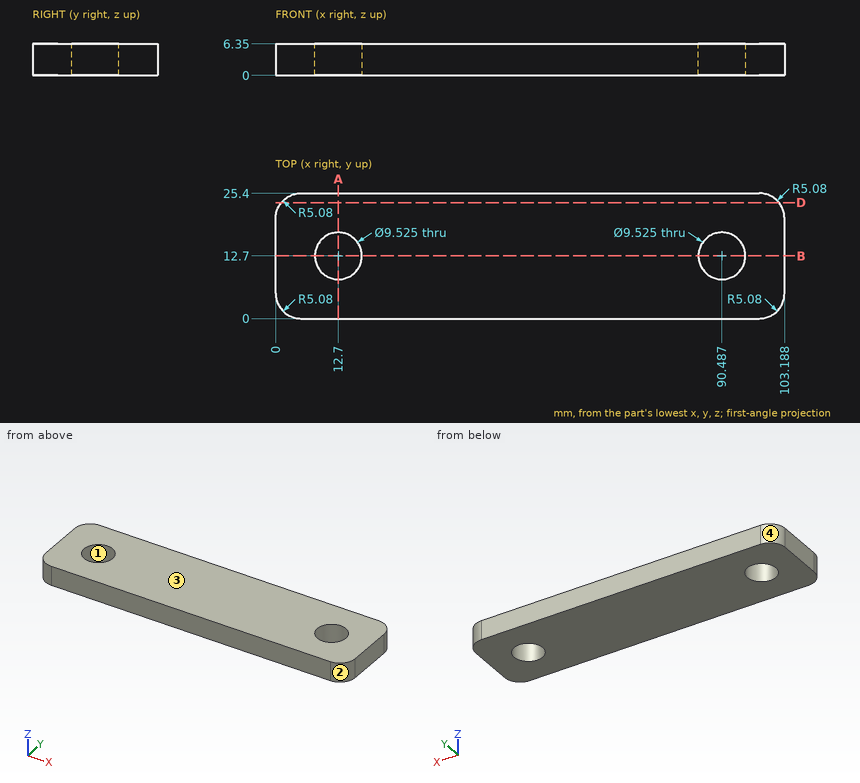
Part print with two shaded views. Sizes in mm from the minimum x, y, z corner. Coordinates: 2 decimals unless noted, no trailing zeros. Order: outer loops, then holes, each group sorted by start corner. A loop starts at its lowest first (then second) coordinate and runs counter-clockwise, first axis right, second up. Notation, with made-up numbers: M 7,3.25 L 36,3.25 A27 ccw 36,37.25 Z; hole C 20,-11 d11. An arc over 180 degrees is marked long. One line per question, with ' | ' between items. Start each with the question number.
1. Cut at B-B (y = 12.7). Count the separate pieces of the cut face and the enclosed holes in it, plus the area to 3 significant figures.
2. Mould opens along Y. For the marked faces 1, 2, 3 and 4 say: +Y half, -Y half, draft (parallel to the pull), parting line (faces both ways), or undercut.
3. Cut at D-D (y = 23.5). Write the cut outline in (x, z).
4. Cut at A-A (x = 12.7). Write the cut outline in (y, z).
5. Wall check: line 1 along X through (y, z) = (13, 4) (1 decimal); line 2 along X through (y, z) = (12.25, 2.75); line 3 along Y through (x, z) = (12.7, 4). Give the ranges that are in metal, low to high. Write a range as [from, to].
The answers:
1) separate pieces: 3 | enclosed holes: 0 | area: 534 mm2
2) face 1: undercut | face 2: -Y half | face 3: draft | face 4: +Y half
3) outline: M 1.12,0 L 102.07,0 L 102.07,6.35 L 1.12,6.35 Z
4) outline: M 0,0 L 7.94,0 L 7.94,6.35 L 0,6.35 Z; M 17.46,0 L 25.4,0 L 25.4,6.35 L 17.46,6.35 Z
5) line 1: x = [0, 7.9], [17.5, 85.7], [95.2, 103.2] | line 2: x = [0, 7.96], [17.44, 85.75], [95.23, 103.19] | line 3: y = [0, 7.94], [17.46, 25.4]
